Input: part model. Units: mm. Frame: model coordinates. Face numbers are marked on the shaded views. Give positions to 0.01 mm unless a question says otherwise; leave off trailing zeros. Write each loop counter-clockwise with the first axis right and the second up, starting at its lowest first coordinate (ties: lowest second). Pieces come first, ordered by that corner, then holes. Notation, with made-up numbers: (-27.5, 64.25) - (5.5, 64.25) arc R16 ccw to (5.5, 85.25) - close; hole circle Ø3 at (-29.75, 77.25). An arc over 180 degrees is marked (long way). Use a Markdown table: item, result. Add a question column.
1. Mould query, pull axis X, two halves, no side actions, for the marked faces 1 and 2. Classes: released by +X, released by -X, zero draft, split by the parting line, or undercut.
2. Pin query (flat end, axial travel): pin 1 (8 mm diameter, centred on x = 50.5, z = -50, fed in from -Y); pin 2 (10 mm diameter, centred on x = 0.5, z = 10.5, fed in from +Y). Return the tip coordinate at first contact, or that it passes through.
3. Section query B-B, the plane z = -11.5. Return loops of the section in (x, y), plus the area to 3 significant figures.
4. Material intervals for probe 1 along X at (y, z) = (4.25, -34.96); probe 2 along Z at (x, y) = (45, 7.75); probe 3 along Z at (x, y) = (2, 3.25), sorted ascending.
5. Section query D-D, the plane x = 1. Return loops of the section in (y, z).
6. Section query C-C, the plane y = 4.5. Return loops of the section in (x, z), plus the area to 3 significant figures.
7. Section query A-A, the plane x = -45. Return loops of the section in (y, z), plus the area to 3 significant figures.
```python
from build123d import *

# Parameters (mm, degrees)
ESBO_O1_W                = 150
ESBO_O1_H                = 150
RESSALTO_EXTRUS_O2_DEPTH = 12.7
CORTE_EXTRUS_O1_DEPTH    = 10
ESBO_O4_W                = 10
ESBO_O4_H                = 10
CORTE_EXTRUS_O2_DEPTH    = 107.823639706
ESBO_O5_R                = 3
CORTE_EXTRUS_O3_DEPTH    = 12.7
FURO_ROSCADO_DE_M83_D    = 6.8


with BuildPart() as part:
    # Esboço1 → Ressalto-extrusão2 (new body)
    with BuildSketch(Plane(origin=(0, 0, 0), x_dir=(1, 0, 0), z_dir=(0, 1, 0))):
        Rectangle(ESBO_O1_W, ESBO_O1_H)
    extrude(amount=RESSALTO_EXTRUS_O2_DEPTH)

    # Esboço2 → Corte-extrusão1 (cut)
    with BuildSketch(Plane(origin=(0, 12.7, 0), x_dir=(1, 0, 0), z_dir=(0, 1, 0))):
        Polygon((10.25, -20.35), (10.25, 20.35), (-10.25, 20.35), (-10.25, -20.35), (-5, -20.35), (-5, -30.35), (5, -30.35), (5, -20.35), align=None)
    extrude(amount=-CORTE_EXTRUS_O1_DEPTH, mode=Mode.SUBTRACT)

    # Esboço4 → Corte-extrusão2 (cut, through all)
    with BuildSketch(Plane(origin=(0, 12.7, 0), x_dir=(1, 0, 0), z_dir=(0, 1, 0))):
        with Locations((0, -35.35)):
            Rectangle(ESBO_O4_W, ESBO_O4_H)
    extrude(amount=-CORTE_EXTRUS_O2_DEPTH, mode=Mode.SUBTRACT)

    # Esboço5 → Corte-extrusão3 (cut)
    with BuildSketch(Plane(origin=(0, 0, 0), x_dir=(-1, 0, 0), z_dir=(0, -1, 0))):
        with Locations(Location((-45, 34.96, 0), (0, 0, 90))):
            Circle(ESBO_O5_R)
        with Locations(Location((45, 34.96, 0), (0, 0, 90))):
            Circle(ESBO_O5_R)
    extrude(amount=-CORTE_EXTRUS_O3_DEPTH, mode=Mode.SUBTRACT)

    # Furo roscado de M83 (through all)
    with Locations(Plane(origin=(0, 12.7, 0), x_dir=(1, 0, 0), z_dir=(0, 1, 0))):
        with Locations((45, 34.96), (-45, 34.96)):
            Hole(FURO_ROSCADO_DE_M83_D / 2)


solid = part.part
```
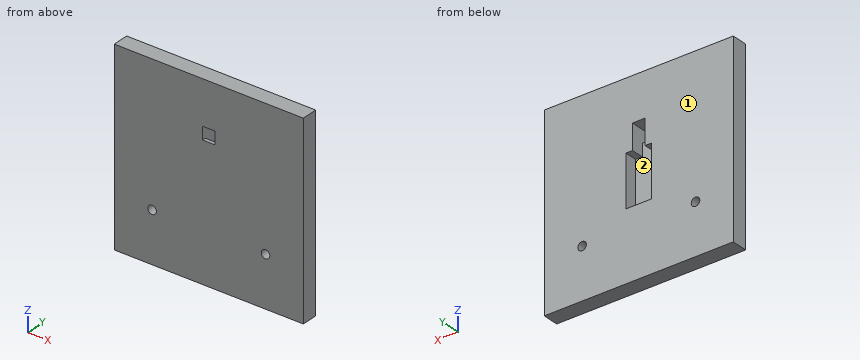
Result sheet:
| question | item | result |
|---|---|---|
| 1 | face 1 | zero draft |
| 1 | face 2 | undercut |
| 2 | pin 1 | stops at y = 0 |
| 2 | pin 2 | stops at y = 2.7 |
| 3 | outline | (-75, 0) - (75, 0) - (75, 12.7) - (10.25, 12.7) - (10.25, 2.7) - (-10.25, 2.7) - (-10.25, 12.7) - (-75, 12.7) - close |
| 3 | area | 1,700 mm² |
| 4 | probe 1 | x = -75 to -48.4, -41.6 to 41.6, 48.4 to 75 |
| 4 | probe 2 | z = -75 to -38.36, -31.56 to 75 |
| 4 | probe 3 | z = -75 to -20.35, 40.35 to 75 |
| 5 | outline | (0, -75) - (12.7, -75) - (12.7, -20.35) - (2.7, -20.35) - (2.7, 30.35) - (0, 30.35) - close; (0, 40.35) - (12.7, 40.35) - (12.7, 75) - (0, 75) - close |
| 6 | outline | (-75, -75) - (75, -75) - (75, 75) - (-75, 75) - close; hole circle Ø6.8 at (-45, -34.96); hole (-10.25, -20.35) - (10.25, -20.35) - (10.25, 20.35) - (5, 20.35) - (5, 40.35) - (-5, 40.35) - (-5, 20.35) - (-10.25, 20.35) - close; hole circle Ø6.8 at (45, -34.96) |
| 6 | area | 21,400 mm² |
| 7 | outline | (0, -75) - (12.7, -75) - (12.7, -38.36) - (0, -38.36) - close; (0, -31.56) - (12.7, -31.56) - (12.7, 75) - (0, 75) - close |
| 7 | area | 1,820 mm² |
